The listing builds one solid part. Answer for the finished solid, in the listing's coordinates (mm). A direction names the side the tool comes from. Give positions to 0.01 mm unless a question says otherwise; leave off trailing zeros. Order: outer loops, then holes, each group sorted by start corner. A loop starts at its lowest first (then second) coordinate and runs counter-clockwise, first axis right, second up. Notation, with made-up numbers: (64.5, -30.5) - (112.5, -30.5) arc R25 cw to (112.5, 8.5) - close; hole circle Ø2 at (31.25, 84). An arc over 180 degrees is marked (long way). Answer as a JSON object with one key per item and string values. Group by question number.
Q1. Given pin 1 (1 mm diameter, centred on x = 8, y = 37.5, fed in from -Z) (3 decimals); pin 2 (1.6 mm diameter, centred on y = -50, z = 31.5, fed in from -X); pin 3 (1 mm diameter, centred on y = -49, z = 28.5, fed in from -X); pin 4 (6 mm diameter, centred on x = -13, z = 18.5, fed in from -Y), each flat-ended and moving along its own axis, determine where each tip first touches the part or whether it passes through.
Q2. A cutting plane is placed at B-B, the plane z = 43.5. Give the vertices of the cut face in (x, y) (3 decimals), and give its area (3 significant figures).
Q3. A cutting plane is placed at A-A, the plane z = 19. Give the vertices of the cut face in (x, y) (1 decimal).
Q4. A cutting plane is placed at C-C, the plane x = 21. Give the vertices of the cut face in (y, z) (3 decimals).
Q5. The mould has two halves that part along X. Classify faces 1 (the face through (-49.351, -49.272, 25.756)), 2 (the face through (46.097, -46.176, 24.146)), 3 (the face through (-1, 1, 50.8)): released by +X, released by -X, zero draft, split by the parting line, or undercut.
Q6. For faces 4 (the face through (49.19, 26.616, 5.878)), 5 (the face through (-34, 49, 38.1)), 6 (the face through (35, -49, 34.925)), 7 (the face through (-47.625, -1, 23)), determine the directions among +Z, -Z, +X, -X, +Y, -Y from which every point of the face is accessible in a straight line to the end or side of a thin tool.
Q7. Consider line 1 (X direction, y = -24, z = 45) (3 decimals); line 2 (Z direction, x = 49.55, y = 25.4). Determine where each line is inside the solid, lowest interval first.
Q8. A cutting plane is placed at D-D, the plane y = 0. Give the vertices of the cut face in (x, z) (1 decimal), and give its area (3 significant figures).
from build123d import *

# Parameters (mm, degrees)
F0_W     = 101.6
F0_H     = 101.6
F0_W_2   = 95.25
F0_H_2   = 95.25
F1_DEPTH = 50.8
F2_DEPTH = 47.625
F3_R     = 5.08
F4_W     = 25.4
F4_H     = 25.4
F4_W_2   = 12.7
F4_H_2   = 12.7
F5_DEPTH = 5.08
F6_W     = 23.495
F6_H     = 38.1
F7_DEPTH = 25.4
F9_D     = 3.3
F9_DEPTH = 6.35
F9_TIP   = 0.9914200214


with BuildPart() as f1:
    # F0 (on Top) → F1 (new body)
    with BuildSketch(Plane.XY):
        Rectangle(F0_W, F0_H)
        Rectangle(F0_W_2, F0_H_2, mode=Mode.SUBTRACT)
        Rectangle(F0_W_2, F0_H_2)
    extrude(amount=F1_DEPTH)

    # F0 (on Top) → F2 (cut)
    with BuildSketch(Plane.XY):
        Rectangle(F0_W_2, F0_H_2)
    extrude(amount=F2_DEPTH, mode=Mode.SUBTRACT)

    # F3
    f3_edges = [f1.edges().sort_by_distance(p)[0] for p in [
        (50.8, -50.8, 25.4),
        (50.8, 50.8, 25.4),
        (-50.8, 50.8, 25.4),
        (-47.625, -47.625, 23.8125),
        (47.625, -47.625, 23.8125),
        (47.625, 47.625, 23.8125),
        (-47.625, 47.625, 23.8125),
        (-50.8, -50.8, 25.4),
    ]]
    fillet(f3_edges, radius=F3_R)

    # F4 (on face) → F5 (cut)
    with BuildSketch(Plane.XZ.offset(50.8)):
        with Locations((-7.9375, 28.575)):
            Rectangle(F4_W, F4_H)
        with Locations((34.925, 28.575)):
            Rectangle(F4_W_2, F4_H_2)
    extrude(amount=-F5_DEPTH, mode=Mode.SUBTRACT)

    # F6 (on face) → F7 (cut)
    with BuildSketch(Plane(origin=(0, 50.8, 0), x_dir=(-1, 0, 0), z_dir=(0, 1, 0))):
        with Locations((33.9725, 19.05)):
            Rectangle(F6_W, F6_H)
    extrude(amount=-F7_DEPTH, mode=Mode.SUBTRACT)

    # F9
    with Locations(Plane.YZ.offset(50.8)):
        with Locations((-25.4, 4.7625), (0, 4.7625), (25.4, 4.7625)):
            Hole(F9_D / 2, depth=F9_DEPTH)
            with Locations((0, 0, -(F9_DEPTH + F9_TIP / 2))):  # 118° drill point
                Cone(0, F9_D / 2, F9_TIP, mode=Mode.SUBTRACT)


solid = f1.part
Reply:
{
 "1": {"pin 1": "stops at z = 47.625", "pin 2": "stops at x = -49.42", "pin 3": "stops at x = -49.97", "pin 4": "stops at y = -50.8"},
 "2": {"outline": "(-50.8, -45.72) arc R5.08 ccw to (-45.72, -50.8) - (45.72, -50.8) arc R5.08 ccw to (50.8, -45.72) - (50.8, 45.72) arc R5.08 ccw to (45.72, 50.8) - (-45.72, 50.8) arc R5.08 ccw to (-50.8, 45.72) - close; hole (-47.625, -42.545) arc R5.08 ccw to (-42.545, -47.625) - (42.545, -47.625) arc R5.08 ccw to (47.625, -42.545) - (47.625, 42.545) arc R5.08 ccw to (42.545, 47.625) - (-42.545, 47.625) arc R5.08 ccw to (-47.625, 42.545) - close", "area": "1,250 mm^2"},
 "3": {"outline": "(-50.8, -45.7) arc R5.1 ccw to (-45.7, -50.8) - (-20.6, -50.8) - (-20.6, -47.6) - (-42.5, -47.6) arc R5.1 cw to (-47.6, -42.5) - (-47.6, 42.5) arc R5.1 cw to (-45.7, 46.5) - (-45.7, 50.8) arc R5.1 ccw to (-50.8, 45.7) - close; (-22.2, 47.6) - (42.5, 47.6) arc R5.1 cw to (47.6, 42.5) - (47.6, -42.5) arc R5.1 cw to (42.5, -47.6) - (4.8, -47.6) - (4.8, -50.8) - (45.7, -50.8) arc R5.1 ccw to (50.8, -45.7) - (50.8, 45.7) arc R5.1 ccw to (45.7, 50.8) - (-22.2, 50.8) - close"},
 "4": {"outline": "(-50.8, 0) - (-47.625, 0) - (-47.625, 47.625) - (47.625, 47.625) - (47.625, 0) - (50.8, 0) - (50.8, 50.8) - (-50.8, 50.8) - close"},
 "5": {"face 1": "released by -X", "face 2": "undercut", "face 3": "zero draft"},
 "6": {"face 4": "+X", "face 5": "-Z, +Y", "face 6": "-Y", "face 7": "-Z"},
 "7": {"line 1": "x = -50.8 to -47.625, 47.625 to 50.8", "line 2": "z = 0 to 3.11, 6.41 to 50.8"},
 "8": {"outline": "(-50.8, 0) - (-47.6, 0) - (-47.6, 47.6) - (47.6, 47.6) - (47.6, 6.4) - (50.8, 6.4) - (50.8, 50.8) - (-50.8, 50.8) - close; (47.6, 0) - (50.8, 0) - (50.8, 3.1) - (47.6, 3.1) - close", "area": "615 mm^2"}
}
